Input: part model. Units: mm. Frame: model coordinates. A direction names the side the tool comes from. Give positions to 0.01 mm unless a question says otherwise; leave off trailing zeros. Write each loop counter-clockwise with the first axis right and the second up, starting at its lowest first coordinate (ties: lowest second). Pieces come first, ordered by that corner, then holes. Notation, with made-up numbers: (-12, -13) -> (8, -13) arc R17 cw to (8, -9) -> close; hole circle Ø10 at (-9.5, 21.25). An arc over 180 degrees is marked (long way). Answer as a JSON object with one key per item and string values. Group by question number.
from build123d import *

# Parameters (mm, degrees)
BOSS_EXTRUDE1_START = 6
SKETCH1_R           = 4
BOSS_EXTRUDE1_DEPTH = 7
BOSS_EXTRUDE2_START = -6
SKETCH1_2_R         = 4
BOSS_EXTRUDE2_DEPTH = 7
SKETCH2_W           = 26
SKETCH2_H           = 16
BOSS_EXTRUDE3_DEPTH = 7
CHAMFER1_SIZE       = 4
SKETCH3_W           = 10
SKETCH3_H           = 8
BOSS_EXTRUDE4_DEPTH = 15
SKETCH5_R           = 4.5
BOSS_EXTRUDE5_DEPTH = 8


with BuildPart() as part:
    # Sketch1 → Boss-Extrude1 (new body)
    with BuildSketch(Plane(origin=(0, 0, 0), x_dir=(0, 0, -1), z_dir=(1, 0, 0)).offset(BOSS_EXTRUDE1_START)):
        with BuildLine():
            Line((8, 10), (-8, 10))
            Line((-8, 10), (-8, 0))
            ThreePointArc((-8, 0), (0, -8), (8, 0))
            Line((8, 0), (8, 10))
        make_face()
        Circle(SKETCH1_R, mode=Mode.SUBTRACT)
    extrude(amount=BOSS_EXTRUDE1_DEPTH)



with BuildPart() as body_2:
    # Sketch1<2> → Boss-Extrude2 (new body)
    with BuildSketch(Plane(origin=(0, 0, 0), x_dir=(0, 0, -1), z_dir=(1, 0, 0)).offset(BOSS_EXTRUDE2_START)):
        with BuildLine():
            Line((8, 10), (-8, 10))
            Line((-8, 10), (-8, 0))
            ThreePointArc((-8, 0), (0, -8), (8, 0))
            Line((8, 0), (8, 10))
        make_face()
        Circle(SKETCH1_2_R, mode=Mode.SUBTRACT)
    extrude(amount=-BOSS_EXTRUDE2_DEPTH)


with BuildPart() as part_1:
    add(part.part)

    add(body_2.part)  # Boss-Extrude3 merges body 2
    # Sketch2 → Boss-Extrude3 (add)
    with BuildSketch(Plane(origin=(0, 10, 0), x_dir=(1, 0, 0), z_dir=(0, 1, 0))):
        Rectangle(SKETCH2_W, SKETCH2_H)
    extrude(amount=BOSS_EXTRUDE3_DEPTH)

    # Chamfer1
    chamfer1_edges = [part_1.edges().sort_by_distance(p)[0] for p in [
        (-13, 17, 0),
        (13, 17, 0),
    ]]
    chamfer(chamfer1_edges, length=CHAMFER1_SIZE)

    # Sketch3 → Boss-Extrude4 (add)
    with BuildSketch(Plane(origin=(0, 17, 0), x_dir=(1, 0, 0), z_dir=(0, 1, 0))):
        Rectangle(SKETCH3_W, SKETCH3_H)
    extrude(amount=BOSS_EXTRUDE4_DEPTH)

    # Sketch5 → Boss-Extrude5 (add, symmetric)
    with BuildSketch(Plane.XY):
        with Locations((0, 26)):
            Circle(SKETCH5_R)
    extrude(amount=BOSS_EXTRUDE5_DEPTH, both=True)


solid = part_1.part
1. Section B-B (y = 26). Return the cut outline in (x, z), plus the area to 3 significant figures.
2. Mould query, pull axis X, two halves, no side actions, for faces 6 (the face through (11, 15, 0)), 7 (the face through (6, 5, 0)), 8 (the face through (-0.59, 30.46, 6.03)). Classes: pulls with the +X half, pulls with the -X half, needs draft (parallel to the pull), parting line crosses it, or undercut.
3. Contact query for flat-ended pins moving along their axis: pin 1 Ø8 at (y, z) = (26.5, 3) entering from -X; pin 2 Ø3 at (x, z) = (-1.5, 6) entering from +Y; pin 3 Ø1 at (x, z) = (-1.5, 6.5) entering from -Y. Output: stop coordinate, or through.
4. Section A-A (z = 0). Return the cut outline in (x, y), plus the area to 3 significant figures.
5. Section D-D (z = 7). Return the cut outline in (x, y).
6. Reachability of faces 1 (the face through (0, 17, -5)), 2 (the face through (0, 26, 8)), 3 (the face through (0, 21, 4)), 4 (the face through (-0.59, 30.46, -5.97)), 5 (the face through (0, 10, 0)) from +Z, -Z, +X, -X, +Y, -Y: full face, straight path, thin tool, end or side. Return the list, or none.
7. Line query: line 1 (X direction, y = 1, z = 6); line 2 (Y direction, x = 3, z = 6.75); line 3 (Z direction, x = 0.5, y = 20.5). Output: solid intervals per line, ascending.
8. Section C-C (x = -10.5). Return the cut outline in (y, z).
Working result:
{
 "1": {"outline": "(-5, -4) -> (-4.5, -4) -> (-4.5, -8) -> (4.5, -8) -> (4.5, -4) -> (5, -4) -> (5, 4) -> (4.5, 4) -> (4.5, 8) -> (-4.5, 8) -> (-4.5, 4) -> (-5, 4) -> close", "area": "152 mm^2"},
 "2": {"face 6": "pulls with the +X half", "face 7": "undercut", "face 8": "parting line crosses it"},
 "3": {"pin 1": "stops at x = -5", "pin 2": "stops at y = 30.5", "pin 3": "stops at y = 10"},
 "4": {"outline": "(-13, -8) -> (-6, -8) -> (-6, -4) -> (-13, -4) -> close; (-13, 4) -> (-6, 4) -> (-6, 10) -> (6, 10) -> (6, 4) -> (13, 4) -> (13, 13) -> (9, 17) -> (5, 17) -> (5, 32) -> (-5, 32) -> (-5, 17) -> (-9, 17) -> (-13, 13) -> close; (6, -8) -> (13, -8) -> (13, -4) -> (6, -4) -> close", "area": "456 mm^2"},
 "5": {"outline": "(-13, -3.87) -> (-6, -3.87) -> (-6, 10) -> (6, 10) -> (6, -3.87) -> (13, -3.87) -> (13, 13) -> (9, 17) -> (-9, 17) -> (-13, 13) -> close; circle Ø9 at (0, 26)"},
 "6": {"face 1": "none", "face 2": "+Z, +X, -X, +Y, -Y", "face 3": "+Z", "face 4": "-Z", "face 5": "+Z, -Z, -Y"},
 "7": {"line 1": "x = -13 to -6, 6 to 13", "line 2": "y = 10 to 17, 22.65 to 29.35", "line 3": "z = -4 to 4"},
 "8": {"outline": "(0, -8) -> (15.5, -8) -> (15.5, 8) -> (0, 8) arc R8 ccw to start; hole circle Ø8 at (0, 0)"}
}
